from build123d import *

# Parameters (mm, degrees)
EXTRUDE_THIN1_DEPTH            = 19.05
SKETCH8_W                      = 15.24
SKETCH8_H                      = 38.1
BOSS_EXTRUDE1_DEPTH            = 12.7
CUT_EXTRUDE1_DEPTH             = 83.853768552
CUT_EXTRUDE1_DEPTH_BACK        = 83.853768552
CUT_EXTRUDE2_REACH             = 79.008
SKETCH10_W                     = 12.954
SKETCH10_H                     = 12.954
CUT_EXTRUDE2_DIRECTION_2_DEPTH = 78.007738646


with BuildPart() as part:
    # Sketch1 → Extrude-Thin1 (new, symmetric)
    with BuildSketch(Plane.XY):
        Polygon((-59.25293848, -13.416886184), (-70.919796031, 0), (-48.877768729, 19.166980263), (-32.21082937, 0), (-34.127527396, -1.666693936), (-49.127772819, 15.583588301), (-67.336404069, -0.25000409), (-57.336240454, -11.750192248), align=None)
    extrude(amount=EXTRUDE_THIN1_DEPTH, both=True)

    # Sketch8 → Boss-Extrude1 (add)
    with BuildSketch(Plane(origin=(-13.869033098, 15.949388063, 0), x_dir=(0.7546055221635044, 0.656178714924787, 0), z_dir=(0.656178714924787, -0.7546055221635044, 0))):
        with Locations((-16.686469716, 0)):
            Rectangle(SKETCH8_W, SKETCH8_H)
    extrude(amount=-BOSS_EXTRUDE1_DEPTH)

    # Sketch9 → Cut-Extrude1 (cut, two sides: drawn at the far end of the back side and taken through both)
    with BuildSketch(Plane(origin=(0, 0, -19.05), x_dir=(-1, 0, 0), z_dir=(0, 0, -1)).offset(-CUT_EXTRUDE1_DEPTH_BACK)):
        Polygon((20.710641212, 10.000163615), (40.544299049, 9.583490131), (29.044110892, 19.583653747), align=None)
    extrude(amount=CUT_EXTRUDE1_DEPTH + CUT_EXTRUDE1_DEPTH_BACK, mode=Mode.SUBTRACT)

    # Sketch10 → Cut-Extrude2 (cut, up to next)
    with BuildSketch(Plane(origin=(-0.21913146, 10.430657518, 0), x_dir=(0.9997793965144279, 0.02100376883433655, 0), z_dir=(-0.02100376883433655, 0.9997793965144279, 0)), mode=Mode.PRIVATE) as cut_extrude2_sk1:
        with Locations((-30.047065424, 0.127)):
            Rectangle(SKETCH10_W, SKETCH10_H)
    cut_extrude2_tool1 = extrude(cut_extrude2_sk1.sketch, amount=-CUT_EXTRUDE2_REACH, mode=Mode.PRIVATE) & part.part
    add(cut_extrude2_tool1.solids().sort_by_distance((-30.259568, 9.799556, -0.127))[0], mode=Mode.SUBTRACT)

    # Sketch10 → Cut-Extrude2 direction 2 (cut)
    with BuildSketch(Plane(origin=(-0.21913146, 10.430657518, 0), x_dir=(0.9997793965144279, 0.02100376883433655, 0), z_dir=(-0.02100376883433655, 0.9997793965144279, 0))):
        with Locations((-30.047065424, 0.127)):
            Rectangle(SKETCH10_W, SKETCH10_H)
    extrude(amount=CUT_EXTRUDE2_DIRECTION_2_DEPTH, mode=Mode.SUBTRACT)


solid = part.part
Read the model definition and answer for the solid it produces. Units are mm, in the model's axes. A direction names the side the tool comes from. Coordinates: 2 decimals unless noted, no trailing zeros. Write each loop counter-clockwise with the first axis right and the second up, starting at its lowest first coordinate (ties: lowest second). Pieces come first, ordered by that corner, then holes. Notation, with made-up numbers: (-35, 0) -> (-3, 0) arc R14 ccw to (-3, 23) -> close; hole circle Ø11 at (43.5, 87.5). An arc over 180 degrees is marked (long way). Return JSON: item names as keys, results as strings.
(1) The part is cut by section C-C on x = -25.5. Give the vertices of the cut face in (y, z), then the cut area to 3 significant figures.
Answers below:
{"outline": "(5.84, -19.05) -> (9.9, -19.05) -> (9.9, -6.6) -> (5.84, -6.6) -> close; (5.84, 6.35) -> (9.9, 6.35) -> (9.9, 19.05) -> (5.84, 19.05) -> close", "area": "102 mm^2"}
(2) Each of these flat-tipped pins is pushed along its axis until it touches: P1, Ø8, axis at x = -45, y = 0, coming from the -Z side; P2, Ø5, axis at y = 4.5, z = -11.5, coming from the -X side; P3, Ø5, axis at y = 2, z = 6.5, coming from the +X side; P4, Ø10, axis at x = -28, z = 6.5, coming from the +Y side. Where does it stop, or does it pass through?
Answers below:
{"P1": "through", "P2": "x = -68.62", "P3": "x = -27.04", "P4": "y = 9.95"}
(3) Consider line 1 along Z through (x, y) = (-35.5, 0.5); line 2 along Y through (x, z) = (-62.5, -2); line 3 along X through (y, z) = (13.5, -11). Determine where each line is inside the solid, lowest interval first. Write a range as from..to.
Answers below:
{"line 1": "-19.05..-6.6, 6.35..19.05", "line 2": "-9.68..-5.81, 3.96..7.32", "line 3": "-55.39..-51.52, -47.32..-43.95"}
(4) Which of the six approach directions +Z, -Z, +X, -X, +Y, -Y give full straight-line access (tool end or side, diameter ignored) to faces 4 (the flat face through (-41.523, 6.838, 0.267)), 5 (the flat face through (-58.1, 7.78, 0.27)), 6 (the flat face through (-42, 8, -19.05))?
Answers below:
{"face 4": "+Z, -Z, -Y", "face 5": "+Z, -Z", "face 6": "-Z, +X, -X, +Y, -Y"}
(5) The part is cut by section B-B on z = -1.5. Give the vertices of the cut face in (x, y), then the cut area to 3 significant figures.
Answers below:
{"outline": "(-70.92, 0) -> (-59.25, -13.42) -> (-57.34, -11.75) -> (-67.34, -0.25) -> (-49.13, 15.58) -> (-36.56, 1.13) -> (-36.74, 9.66) -> (-40.54, 9.58) -> (-48.88, 19.17) -> close; (-23.78, 9.94) -> (-23.73, 7.37) -> (-20.71, 10) -> close", "area": "170 mm^2"}
(6) The part is cut by section A-A on y = 8.5. Give the vertices of the cut face in (x, z), then the cut area to 3 significant figures.
Answers below:
{"outline": "(-61.14, -19.05) -> (-57.27, -19.05) -> (-57.27, 19.05) -> (-61.14, 19.05) -> close; (-42.97, -19.05) -> (-22.44, -19.05) -> (-22.44, 19.05) -> (-42.97, 19.05) -> close; hole (-36.71, -6.6) -> (-23.75, -6.6) -> (-23.75, 6.35) -> (-36.71, 6.35) -> close", "area": "762 mm^2"}
(7) The part is cut by section D-D on z = 8. Give the vertices of the cut face in (x, y).
Answers below:
{"outline": "(-70.92, 0) -> (-59.25, -13.42) -> (-57.34, -11.75) -> (-67.34, -0.25) -> (-49.13, 15.58) -> (-34.13, -1.67) -> (-20.71, 10) -> (-40.54, 9.58) -> (-48.88, 19.17) -> close"}
(8) For a pull along Y with two mould halves and no side action, classify faces 1 (the flat face through (-62.406, -5.92, 0.267)), 2 (the flat face through (-44.77, 14.44, 0.27)), 3 (the flat face through (-65.005, -6.802, 0.267)) as pulls with the +Y half, pulls with the -Y half, needs draft (parallel to the pull), parting line crosses it, or undercut.
Answers below:
{"face 1": "undercut", "face 2": "pulls with the +Y half", "face 3": "pulls with the -Y half"}
